Design review of the part built by this model. Coordinates are the model's own, in mm. A direction names the side the tool comes from. Round coordinates to 2 decimals unless told otherwise and drop trailing zeros. Loops run counter-clockwise (first coordinate to the right, second up) from the corner with the lowest first, then second, coordinate; pieces in that order, holes last. Notation, with made-up numbers: M 73.5,68 L 103.5,68 A25 cw 103.5,105 Z; hole C 41.5,81 d2. An arc over 180 degrees is marked long. Use a Markdown table: item, result.
from build123d import *

# Parameters (mm, degrees)
SKETCH1_R           = 20
BOSS_EXTRUDE1_DEPTH = 8
SKETCH2_R           = 16
CUT_EXTRUDE1_DEPTH  = 6.35
SKETCH3_W           = 5
SKETCH3_H           = 6.35
BOSS_EXTRUDE2_DEPTH = 3
CUT_EXTRUDE2_DEPTH  = 177.8


with BuildPart() as part:
    # Sketch1 → Boss-Extrude1 (new body)
    with BuildSketch(Plane.XY):
        Circle(SKETCH1_R)
    extrude(amount=BOSS_EXTRUDE1_DEPTH)

    # Sketch2 → Cut-Extrude1 (cut)
    with BuildSketch(Plane(origin=(0, 0, 0), x_dir=(-1, 0, 0), z_dir=(0, 0, -1))):
        Circle(SKETCH2_R)
    extrude(amount=-CUT_EXTRUDE1_DEPTH, mode=Mode.SUBTRACT)

    # Sketch3 → Boss-Extrude2 (add)
    with BuildSketch(Plane.XY.offset(8)):
        with Locations((-5, -3.175)):
            Rectangle(SKETCH3_W, SKETCH3_H)
        with Locations((-5, 3.175)):
            Rectangle(SKETCH3_W, SKETCH3_H)
        with Locations((5, 3.175)):
            Rectangle(SKETCH3_W, SKETCH3_H)
        with Locations((5, -3.175)):
            Rectangle(SKETCH3_W, SKETCH3_H)
    extrude(amount=BOSS_EXTRUDE2_DEPTH)

    # Sketch6 → Cut-Extrude2 (cut)
    with BuildSketch(Plane.ZY.offset(7.5)):
        Polygon((10.05, -5.35), (10.05, -2.328333333), (8.95, 2.328333333), (8.95, -5.35), align=None)
        Polygon((8.95, 2.328333333), (10.05, -2.328333333), (10.05, 5.35), (8.95, 5.35), align=None)
    extrude(amount=-CUT_EXTRUDE2_DEPTH, mode=Mode.SUBTRACT)


solid = part.part
1. Take a section at D-D on z = 5. Give the boundary of the cut face in (x, y).
Check values:
| item | result |
|---|---|
| outline | C 0,0 d40; hole C 0,0 d32 |
2. Wall thickness on line 1 along Y through (x, z) = (0, 1.5); line 2 along Z through (x, y) = (2.5, 11); line 3 along Z through (x, y) = (-6, 0): over which ranges is each line inside the solid? List them lowest first. Write a range as from..to.
Check values:
| item | result |
|---|---|
| line 1 | y = -20..-16, 16..20 |
| line 2 | z = 6.35..8 |
| line 3 | z = 6.35..8.95, 10.05..11 |
3. Insertion check: pin 1 (2 mm diameter, centred on y = -2, z = 8.5, fed in from -X); pin 2 (2.5 mm diameter, centred on x = 4.5, z = 10, fed in from +Y); pin 3 (0.9 mm diameter, centred on y = -1, z = 9, fed in from -X). Each pin has a flat end and moves straight along its axis. Give the tip position at first contact, or say it passes through.
Check values:
| item | result |
|---|---|
| pin 1 | stops at x = -19.97 |
| pin 2 | stops at y = 6.35 |
| pin 3 | stops at x = -7.5 |
4. Take a section at B-B on x = 0. Give the boundary of the cut face in (y, z).
Check values:
| item | result |
|---|---|
| outline | M -20,0 L -16,0 L -16,6.35 L 16,6.35 L 16,0 L 20,0 L 20,8 L -20,8 Z |
5. The part is to be moulded in two halves that separate along Y. For faces 6 (the face through (-5, 0, 8.95)), 7 (the face through (-5, -5.35, 9.5)), 8 (the face through (-5, 0, 11)), 9 (the face through (5, 6.35, 9)), say which applies: pulls with the +Y half, pulls with the -Y half, needs draft (parallel to the pull), parting line crosses it, or undercut.
Check values:
| item | result |
|---|---|
| face 6 | undercut |
| face 7 | undercut |
| face 8 | needs draft |
| face 9 | pulls with the +Y half |
6. Take a section at A-A on y = 0. Give the boundary of the cut face in (x, z).
Check values:
| item | result |
|---|---|
| outline | M -20,0 L -16,0 L -16,6.35 L 16,6.35 L 16,0 L 20,0 L 20,8 L 7.5,8 L 7.5,8.95 L 2.5,8.95 L 2.5,8 L -2.5,8 L -2.5,8.95 L -7.5,8.95 L -7.5,8 L -20,8 Z; M -7.5,10.05 L -2.5,10.05 L -2.5,11 L -7.5,11 Z; M 2.5,10.05 L 7.5,10.05 L 7.5,11 L 2.5,11 Z |
7. Machinability: for faces 1 (the face through (3.47, -15.62, 3.13)), 2 (the face through (5, -6.35, 9)), 3 (the face through (2.5, 0.1, 10.5)), 4 (the face through (5, 0, 10.05)), 5 (the face through (-7.5, 0.1, 10.5)), which of the approach directions +Z, -Z, +X, -X, +Y, -Y give a long, thin tool a straight path to every point of the face, cutting with its end or side? Answer none if there is none.
Check values:
| item | result |
|---|---|
| face 1 | -Z |
| face 2 | +Z, +X, -X, -Y |
| face 3 | +Z, +Y, -Y |
| face 4 | +X, -X |
| face 5 | +Z, -X, +Y, -Y |
8. Take a section at C-C on y = 15. Give the boundary of the cut face in (x, z), and give its area (3 significant figures).
Check values:
| item | result |
|---|---|
| outline | M -13.23,0 L -5.57,0 L -5.57,6.35 L 5.57,6.35 L 5.57,0 L 13.23,0 L 13.23,8 L -13.23,8 Z |
| area | 141 mm² |
